```python
from build123d import *

# Parameters (mm, degrees)
SKETCH1_W              = 365
SKETCH1_H              = 300
BOSS_EXTRUDE1_DEPTH    = 16
SKETCH2_W              = 365
SKETCH2_H              = 16
BOSS_EXTRUDE2_DEPTH    = 200
BOSS_EXTRUDE3_START    = -69.5
BOSS_EXTRUDE3_DEPTH    = 16
BOSS_EXTRUDE4_START    = 194
BOSS_EXTRUDE4_DEPTH    = 16
M8X1_25_TAPPED_HOLE1_D = 6.8
LPATTERN1_COUNT        = 2
LPATTERN1_PITCH        = 335


with BuildPart() as part:
    # Sketch1 → Boss-Extrude1 (new body)
    with BuildSketch(Plane.XY):
        with Locations((0, -150)):
            Rectangle(SKETCH1_W, SKETCH1_H)
    extrude(amount=BOSS_EXTRUDE1_DEPTH)

    # Sketch2 → Boss-Extrude2 (add)
    with BuildSketch(Plane.XY.offset(16)):
        with Locations((0, -8)):
            Rectangle(SKETCH2_W, SKETCH2_H)
    extrude(amount=BOSS_EXTRUDE2_DEPTH)

    # Sketch3 → Boss-Extrude3 (add)
    with BuildSketch(Plane(origin=(182.5, 0, 0), x_dir=(0, 0, -1), z_dir=(1, 0, 0)).offset(BOSS_EXTRUDE3_START)):
        Polygon((-216, -16), (-216, -66), (-65.197290638, -300), (-16, -300), (-16, -16), align=None)
    extrude(amount=-BOSS_EXTRUDE3_DEPTH)

    # Sketch4 → Boss-Extrude4 (add)
    with BuildSketch(Plane.ZY.offset(-97).offset(BOSS_EXTRUDE4_START)):
        Polygon((216, -16), (16, -16), (16, -300), (65.197290638, -300), (216, -66), align=None)
    extrude(amount=BOSS_EXTRUDE4_DEPTH)

    # M8x1.25 Tapped Hole1 (through all)
    with Locations(Plane.XY.offset(16)):
        with Locations((167.5, -30), (167.5, -270), (167.5, -198), (167.5, -102)):
            m8x1_25_tapped_hole1 = Hole(M8X1_25_TAPPED_HOLE1_D / 2)

    # LPattern1: M8x1.25 Tapped Hole1 ×2
    with Locations(*[(-i * LPATTERN1_PITCH, 0, 0) for i in range(1, LPATTERN1_COUNT)]):
        add(m8x1_25_tapped_hole1, mode=Mode.SUBTRACT)


solid = part.part
```
The listing builds one solid part. Answer for the finished solid, in the listing's coordinates (mm). A direction names the side the tool comes from. Round coordinates to 2 decimals unless told otherwise and drop trailing zeros. Write each loop counter-clockwise with the first axis right and the second up, starting at its lowest first coordinate (ties: lowest second). Pieces come first, ordered by that corner, then holes. Notation, with made-up numbers: (-25, 16.25) -> (8, 16.25) arc R31 ccw to (8, 49.25) -> close; hole circle Ø4 at (-38.5, -15). An arc over 180 degrees is marked (long way). Use CSV: the item, a comma, the result in double quotes. Start each with the question number.
(1) Section A-A on z = 41 is taken. Give the vertices of the cut face in (x, y).
(2) Section C-C on y = -189.5 is taken. Give the vertices of the cut face in (x, z), then the cut area to 3 significant figures.
(3) Each of these flat-tipped pins is pushed along its axis until it touches: pin 1 (3 mm diameter, centred on y = -80, z = 110, fed in from -X); pin 2 (5.5 mm diameter, centred on x = -167.5, y = -270, fed in from +Z); pin 3 (12 mm diameter, centred on x = -26.5, y = -76, fed in from +Z); pin 4 (10 mm diameter, centred on x = 2, z = 174, fed in from -Y). Where does it stop, or does it pass through?
(4) Which of the six approach directions +Z, -Z, +X, -X, +Y, -Y give full straight-line access (tool end or side, diameter ignored) to faces 4 (the face through (147, -156, 16)), 5 (the face through (97, -124, 95)), 6 (the face through (-104.89, -184.64, 139.54)), 7 (the face through (-148, -156, 16))?
(5) Consider L1, parallel to Y at x = 167.5, z = 11; L2, parallel to X at y = -198, z = 11.25; L3, parallel to X at y = -192, z = 24. Determine where each line is inside the solid, lowest interval first. Write a range as from..to.
(6) Section B-B on x = 31 is taken. Give the vertices of the cut face in (y, z), then the cut area to 3 significant figures.
(7) The mould has two halves that part along X. Classify faces 1 (the face through (182.5, -106, 11)), 2 (the face through (147, -16, 115)), 3 (the face through (-1, -16, 115)): released by +X, released by -X, zero draft, split by the parting line, or undercut.
A:
1,outline,"(-182.5, -16) -> (-113, -16) -> (-113, -300) -> (-97, -300) -> (-97, -16) -> (97, -16) -> (97, -300) -> (113, -300) -> (113, -16) -> (182.5, -16) -> (182.5, 0) -> (-182.5, 0) -> close"
2,outline,"(-182.5, 0) -> (182.5, 0) -> (182.5, 16) -> (113, 16) -> (113, 136.41) -> (97, 136.41) -> (97, 16) -> (-97, 16) -> (-97, 136.41) -> (-113, 136.41) -> (-113, 16) -> (-182.5, 16) -> close"
2,area,"9,690 mm²"
3,pin 1,"stops at x = -113"
3,pin 2,"passes through"
3,pin 3,"stops at z = 16"
3,pin 4,"stops at y = -16"
4,face 4,"+Z, +X, -Y"
4,face 5,"+Z, -Y"
4,face 6,"+Z, +X, -X, -Y"
4,face 7,"+Z, -X, -Y"
5,L1,"y = -300..-273.4, -266.6..-201.4, -194.6..-105.4, -98.6..-33.4, -26.6..0"
5,L2,"x = -182.5..-170.9, -164.1..164.1, 170.9..182.5"
5,L3,"x = -113..-97, 97..113"
6,outline,"(-300, 0) -> (0, 0) -> (0, 216) -> (-16, 216) -> (-16, 16) -> (-300, 16) -> close"
6,area,"8,000 mm²"
7,face 1,"released by +X"
7,face 2,"zero draft"
7,face 3,"undercut"
